from build123d import *

# Parameters (mm, degrees)
SKETCH1_W                             = 100
SKETCH1_H                             = 100
SKETCH1_R                             = 32
BOSS_EXTRUDE3_DEPTH                   = 6.35
M4_CLEARANCE_HOLE2_D                  = 4.5
M4_CLEARANCE_HOLE2_CSINK_D            = 4.55
M4_CLEARANCE_HOLE2_CSINK_ANGLE        = 90
TAP_DRILL_FOR_M3X0_5_TAP2_D           = 2.5
TAP_DRILL_FOR_M3X0_5_TAP2_DEPTH       = 9.248924226
TAP_DRILL_FOR_M3X0_5_TAP2_CSINK_D     = 2.55
TAP_DRILL_FOR_M3X0_5_TAP2_CSINK_ANGLE = 90
TAP_DRILL_FOR_M3X0_5_TAP2_TIP         = 0.751075774
SKETCH32_W                            = 100
SKETCH32_H                            = 6.35
CUT_EXTRUDE1_DEPTH                    = 10
TAP_DRILL_FOR_M3X0_5_TAP4_D           = 2.5
TAP_DRILL_FOR_M3X0_5_TAP4_DEPTH       = 9.248924226
TAP_DRILL_FOR_M3X0_5_TAP4_CSINK_D     = 2.55
TAP_DRILL_FOR_M3X0_5_TAP4_CSINK_ANGLE = 90
TAP_DRILL_FOR_M3X0_5_TAP4_TIP         = 0.751075774
SKETCH36_W                            = 5.7
SKETCH36_H                            = 2.6
CUT_EXTRUDE2_DEPTH                    = 71.995228713


with BuildPart() as part:
    # Sketch1 → Boss-Extrude3 (new body)
    with BuildSketch(Plane(origin=(0, 0, 0), x_dir=(1, 0, 0), z_dir=(0, 1, 0))):
        Rectangle(SKETCH1_W, SKETCH1_H)
        with Locations(Location((0, 0, 0), (0, 0, 270))):
            Circle(SKETCH1_R, mode=Mode.SUBTRACT)
    extrude(amount=BOSS_EXTRUDE3_DEPTH)

    # M4 Clearance Hole2 (through all)
    with Locations(Plane(origin=(0, 0, 0), x_dir=(-1, 0, 0), z_dir=(0, -1, 0))):
        with Locations((-9.188076101, 34.290366833), (25.102290732, 25.102290732), (34.290366833, -9.188076101), (9.188076101, -34.290366833), (-25.102290732, -25.102290732), (-34.290366833, 9.188076101)):
            CounterSinkHole(M4_CLEARANCE_HOLE2_D / 2, M4_CLEARANCE_HOLE2_CSINK_D / 2, counter_sink_angle=M4_CLEARANCE_HOLE2_CSINK_ANGLE)

    # Tap Drill for M3x0.5 Tap2
    with Locations(Plane.XY.offset(50)):
        with Locations((-35, 3.175), (35, 3.175)):
            CounterSinkHole(TAP_DRILL_FOR_M3X0_5_TAP2_D / 2, TAP_DRILL_FOR_M3X0_5_TAP2_CSINK_D / 2, depth=TAP_DRILL_FOR_M3X0_5_TAP2_DEPTH, counter_sink_angle=TAP_DRILL_FOR_M3X0_5_TAP2_CSINK_ANGLE)
            with Locations((0, 0, -(TAP_DRILL_FOR_M3X0_5_TAP2_DEPTH + TAP_DRILL_FOR_M3X0_5_TAP2_TIP / 2))):  # 118° drill point
                Cone(0, TAP_DRILL_FOR_M3X0_5_TAP2_D / 2, TAP_DRILL_FOR_M3X0_5_TAP2_TIP, mode=Mode.SUBTRACT)

    # Sketch32 → Cut-Extrude1 (cut)
    with BuildSketch(Plane(origin=(0, 6.35, 0), x_dir=(1, 0, 0), z_dir=(0, 1, 0))):
        with Locations((0, 46.825)):
            Rectangle(SKETCH32_W, SKETCH32_H)
    extrude(amount=-CUT_EXTRUDE1_DEPTH, mode=Mode.SUBTRACT)

    # Tap Drill for M3x0.5 Tap4
    with Locations(Plane(origin=(0, 0, -43.65), x_dir=(-1, 0, 0), z_dir=(0, 0, -1))):
        with Locations((-35, 3.175), (35, 3.175)):
            CounterSinkHole(TAP_DRILL_FOR_M3X0_5_TAP4_D / 2, TAP_DRILL_FOR_M3X0_5_TAP4_CSINK_D / 2, depth=TAP_DRILL_FOR_M3X0_5_TAP4_DEPTH, counter_sink_angle=TAP_DRILL_FOR_M3X0_5_TAP4_CSINK_ANGLE)
            with Locations((0, 0, -(TAP_DRILL_FOR_M3X0_5_TAP4_DEPTH + TAP_DRILL_FOR_M3X0_5_TAP4_TIP / 2))):  # 118° drill point
                Cone(0, TAP_DRILL_FOR_M3X0_5_TAP4_D / 2, TAP_DRILL_FOR_M3X0_5_TAP4_TIP, mode=Mode.SUBTRACT)

    # Sketch36 → Cut-Extrude2 (cut, through all)
    with BuildSketch(Plane(origin=(0, 6.35, 0), x_dir=(1, 0, 0), z_dir=(0, 1, 0))):
        with Locations((-35, -46.2)):
            Rectangle(SKETCH36_W, SKETCH36_H)
        with Locations((35, -46.2)):
            Rectangle(SKETCH36_W, SKETCH36_H)
        with Locations((35, 39.825)):
            Rectangle(SKETCH36_W, SKETCH36_H)
        with Locations((-35, 39.825)):
            Rectangle(SKETCH36_W, SKETCH36_H)
    extrude(amount=-CUT_EXTRUDE2_DEPTH, mode=Mode.SUBTRACT)


solid = part.part
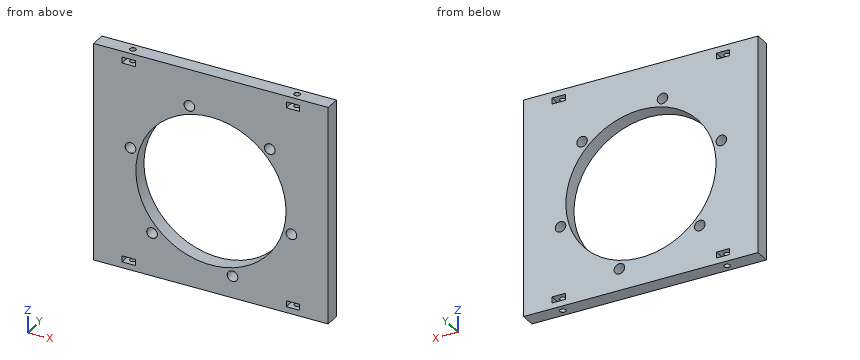
The listing builds one solid part. Answer for the finished solid, in the listing's coordinates (mm). Coordinates: 2 decimals unless noted, no trailing zeros. Write each loop counter-clockwise with the first axis right and the second up, starting at its lowest first coordinate (ties: lowest second). Pieces come first, ordered by that corner, then holes. Notation, with made-up numbers: (43, -4.5) - (92, -4.5) arc R7 ccw to (92, 6.5) - close; hole circle Ø9 at (86, 83). An arc over 180 degrees is marked (long way). Put each result on its own line as item: value.
1. The part is cut by section A-A on z = 0. Give the vertices of the cut face in (x, y), plus the area to 3 significant figures.
Answer sheet:
outline: (-50, 0) - (-32, 0) - (-32, 6.35) - (-50, 6.35) - close; (32, 0) - (50, 0) - (50, 6.35) - (32, 6.35) - close
area: 229 mm^2
2. Flat-ended cylindrical pins translate along their axes: pin 1 Ø1.5 at (x, y) = (35, 3.175) entering from +Z; pin 2 Ø1.5 at (x, y) = (-35, 3.175) entering from -Z. Find the tip coordinate at first contact, or state that the pin passes through.
Answer sheet:
pin 1: stops at z = 40.45
pin 2: stops at z = -34.1
3. Find the intervals of material crossed by line 1 along Y through (x, z) = (-35, -42.7) (3 decimals); line 2 along X through (y, z) = (4.5, 0); line 3 along Z through (x, y) = (26, 1.75), in increasing order. Write a range as from..to.
Answer sheet:
line 1: y = 0..1.925, 4.425..6.35
line 2: x = -50..-32, 32..50
line 3: z = -43.65..-18.65, 18.65..23.04, 27.17..50
4. The part is cut by section B-B on x = 0. Give the vertices of the cut face in (y, z).
Answer sheet:
outline: (0, -43.65) - (6.35, -43.65) - (6.35, -32) - (0, -32) - close; (0, 32) - (6.35, 32) - (6.35, 50) - (0, 50) - close
